from build123d import *

# Parameters (mm, degrees)
SKETCH1_W           = 144
SKETCH1_H           = 20
BOSS_EXTRUDE1_DEPTH = 6
HOLE1_AT_2_COUNT    = 2
HOLE1_AT_2_PITCH    = 70


with BuildPart() as part:
    # Sketch1 → Boss-Extrude1 (new body)
    with BuildSketch(Plane(origin=(0, 0, 0), x_dir=(1, 0, 0), z_dir=(0, 1, 0))):
        Rectangle(SKETCH1_W, SKETCH1_H)
    extrude(amount=BOSS_EXTRUDE1_DEPTH)

    # Sketch3 → Hole1 (revolve, cut)
    with BuildSketch(Plane(origin=(-35, 6, 0), x_dir=(0, 0, 1), z_dir=(1, 0, 0))):
        Polygon((0, 0), (0, 6), (3.2, 6), (3.2, 3.1), (6.3, 0), align=None)
    hole1 = revolve(axis=Axis((-35, 20.308894879, 0), (0, -1, 0)), mode=Mode.SUBTRACT)

    # Hole1 at 2: Hole1 ×2
    with Locations(*[(i * HOLE1_AT_2_PITCH, 0, 0) for i in range(1, HOLE1_AT_2_COUNT)]):
        add(hole1, mode=Mode.SUBTRACT)


solid = part.part
Verification items for the finished model (mm, model axes). Coordinates: 2 decimals unless noted, no trailing zeros. Order: outer loops, then holes, each group sorted by start corner. A loop starts at its lowest first (then second) coordinate and runs counter-clockwise, first axis right, second up. Notation, with made-up numbers: M -26,79 L 0,79 A22 cw 0,92 Z; hole C -23.5,-0.75 d6. An arc over 180 degrees is marked long. One line per item, written item: value. Start each with the question number.
Item 1: Scan lines: probe 1 along X at (y, z) = (1.5, 0); probe 2 along Z at (x, y) = (-35, 1.25); probe 3 along X at (y, z) = (4.7, 3.25). Record each from-to range of solid material in increasing order.
Item 2: Gauge pin test, flat end, axial feed: pin 1 (8.5 mm diameter, centred on x = -35, z = 0, fed in from +Y). Record the tip position at first contact, or that the pin passes through.
Item 3: Sectioned sample at C-C (y = 4.55). Enter the section's corners in (x, z), then the cut area to 3 significant figures.
Item 4: Sectioned sample at A-A (z = 0). Enter the section's corners in (x, y), then the cut area to 3 significant figures.
Item 5: Mould release check, pull along X, two halves, no side actions. Record for faces 1 (the flat face through (-1, 3, -10)), 2 (the cylindrical face through (31.827, 1.47, -0.417)), 3 (the flat face through (72, 3, 0)), 4 (the cylindrical face through (-38.173, 1.47, -0.417)): released by +X, released by -X, zero draft, split by the parting line, or undercut.
Item 6: Sectioned sample at B-B (x = 35). Enter the section's corners in (y, z).
Conclusion:
1. probe 1: x = -72 to -38.2, -31.8 to 31.8, 38.2 to 72
1. probe 2: z = -10 to -3.2, 3.2 to 10
1. probe 3: x = -72 to -38.8, -31.2 to 31.2, 38.8 to 72
2. pin 1: stops at y = 3.95
3. outline: M -72,-10 L 72,-10 L 72,10 L -72,10 Z; hole C -35,0 d9.7; hole C 35,0 d9.7
3. area: 2,730 mm^2
4. outline: M -72,0 L -38.2,0 L -38.2,2.9 L -41.3,6 L -72,6 Z; M -31.8,0 L 31.8,0 L 31.8,2.9 L 28.7,6 L -28.7,6 L -31.8,2.9 Z; M 38.2,0 L 72,0 L 72,6 L 41.3,6 L 38.2,2.9 Z
4. area: 768 mm^2
5. face 1: zero draft
5. face 2: undercut
5. face 3: released by +X
5. face 4: undercut
6. outline: M 0,-10 L 6,-10 L 6,-6.3 L 2.9,-3.2 L 0,-3.2 Z; M 0,3.2 L 2.9,3.2 L 6,6.3 L 6,10 L 0,10 Z
